Verification items for the finished model (mm, model axes). Coordinates: 2 decimals unless noted, no trailing zeros. Order: outer loops, then holes, each group sorted by start corner. A loop starts at its lowest first (then second) coordinate and runs counter-clockwise, first axis right, second up. Notation, with made-up numbers: M 81,48 L 130,48 A18 cw 130,73 Z; hole C 25,-11 d9. An arc over 180 degrees is marked long. Return JSON: item names as keys, results as strings.
```python
from build123d import *

# Parameters (mm, degrees)
F1_DEPTH = 7


with BuildPart() as f1:
    # F0 (on Top) → F1 (new body)
    with BuildSketch(Plane.XY):
        with BuildLine():
            Line((6, -12), (6, 12))
            Line((6, 12), (4.038874, 12))
            ThreePointArc((4.038874, 12), (4.568761, 10.799587), (4.75, 9.5))
            ThreePointArc((4.75, 9.5), (-1.299587, 4.931239), (-4.038874, 12))
            Line((-4.038874, 12), (-6, 12))
            Line((-6, 12), (-6, -12))
            Line((-6, -12), (-4.038874, -12))
            ThreePointArc((-4.038874, -12), (-1.299587, -4.931239), (4.75, -9.5))
            ThreePointArc((4.75, -9.5), (4.568761, -10.799587), (4.038874, -12))
            Line((4.038874, -12), (6, -12))
        make_face()
    extrude(amount=F1_DEPTH)


solid = f1.part
```
Q1. Cross-section at A-A, the plane y = -9.25. Record the boundary of the cut face in (x, z), and give its area (3 significant figures).
Values:
{"outline": "M -6,0 L -4.74,0 L -4.74,7 L -6,7 Z; M 4.74,0 L 6,0 L 6,7 L 4.74,7 Z", "area": "17.6 mm^2"}
Q2. Cross-section at C-C, the plane y = 10.5. Record the boundary of the cut face in (x, z), and give its area (3 significant figures).
Values:
{"outline": "M -6,0 L -4.64,0 L -4.64,7 L -6,7 Z; M 4.64,0 L 6,0 L 6,7 L 4.64,7 Z", "area": "19.0 mm^2"}
Q3. Cross-section at B-B, the plane z = 3.25. Record the boundary of the cut face in (x, y).
Values:
{"outline": "M -6,-12 L -4.04,-12 A4.75 cw long 4.75,-9.5 A4.75 cw 4.04,-12 L 6,-12 L 6,12 L 4.04,12 A4.75 cw 4.75,9.5 A4.75 cw long -4.04,12 L -6,12 Z"}
Q4. Material ranges on line 1 along X through (y, z) = (-9.5, 4.75); line 2 along Y through (x, z) = (-4.25, 3.5); line 3 along Y through (x, z) = (0, 5.75), recorded low to high.
Values:
{"line 1": "-6 to -4.75, 4.75 to 6", "line 2": "-12 to -11.62, -7.38 to 7.38, 11.62 to 12", "line 3": "-4.75 to 4.75"}
Q5. Cross-section at D-D, the plane x = 1. Record the boundary of the cut face in (y, z).
Values:
{"outline": "M -4.86,0 L 4.86,0 L 4.86,7 L -4.86,7 Z"}
Q6. Go/stop test with flat-tipped pins: pin 1 (2 mm diameter, centred on x = 2.5, z = 3, fed in from -Y); pin 2 (1 mm diameter, centred on x = 1.5, z = 1.5, fed in from +Y). Record where each tip stops, or that it passes through.
Values:
{"pin 1": "y = -6.29", "pin 2": "y = 5.19"}
